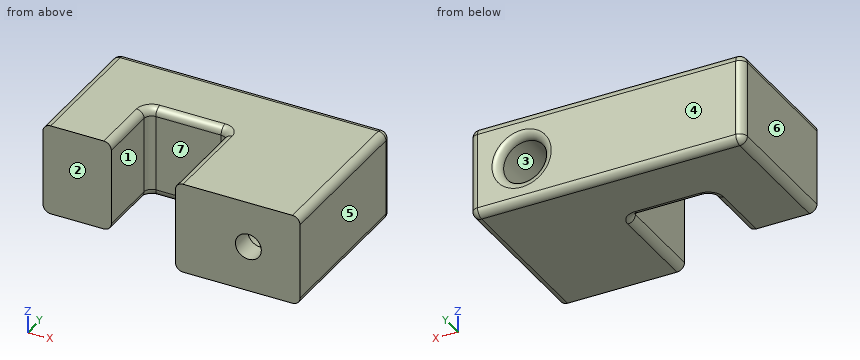
```python
from build123d import *

# Parameters (mm, degrees)
F1_DEPTH = 15.24
F2_R     = 2.159
F3_DEPTH = 27.94
F4_R     = 3.683
F5_DEPTH = 24.13
F6_F1_R  = 1.27
F6_F2_R  = 1.27
F6_F3_R  = 1.27


with BuildPart() as f1:
    # F0 (on Top) → F1 (new body)
    with BuildSketch(Plane.XY):
        Polygon((-11.43, 0), (0, 0), (0, 11.43), (13.462, 11.43), (13.462, -5.08), (34.29, -5.08), (34.29, 22.86), (-11.43, 22.86), align=None)
    extrude(amount=F1_DEPTH)

    # F2 (on face) → F3 (cut, through all)
    with BuildSketch(Plane.XZ.offset(5.08)):
        with Locations((25.654, 7.62)):
            Circle(F2_R)
    extrude(amount=-F3_DEPTH, mode=Mode.SUBTRACT)

    # F4 (on face) → F5 (cut)
    with BuildSketch(Plane(origin=(0, 22.86, 0), x_dir=(-1, 0, 0), z_dir=(0, 1, 0))):
        with Locations((-25.654, 7.62)):
            Circle(F4_R)
    extrude(amount=-F5_DEPTH, mode=Mode.SUBTRACT)

    # F6: fillet of radius 1.27 on 14 edges, made by hand

    # F6_f1
    f6_f1_edges = [f1.edges().sort_by_distance(p)[0] for p in [
        (0, 11.43, 7.62),
        (13.462, 11.43, 7.62),
    ]]
    fillet(f6_f1_edges, radius=F6_F1_R)

    # F6_f2
    f6_f2_edges = [f1.edges().sort_by_distance(p)[0] for p in [
        (6.731, 11.43, 15.24),
        (-11.43, 22.86, 7.62),
        (-11.43, 11.43, 15.24),
        (-11.43, 11.43, 0),
        (11.43, 22.86, 15.24),
        (34.29, 22.86, 7.62),
        (34.29, 8.89, 15.24),
        (34.29, 8.89, 0),
        (11.43, 22.86, 0),
        (29.337, 22.86, 7.62),
        (0.3719743879, 11.0580256121, 15.24),
        (13.0900256121, 11.0580256121, 15.24),
    ]]
    fillet(f6_f2_edges, radius=F6_F2_R)

    # F6_f3
    f6_f3_edges = [f1.edges().sort_by_distance(p)[0] for p in [
        (0, 5.08, 0),
        (6.731, 11.43, 0),
        (0.3719743879, 11.0580256121, 0),
        (13.0900256121, 11.0580256121, 0),
    ]]
    fillet(f6_f3_edges, radius=F6_F3_R)


solid = f1.part
```
Can you work these out from the model? Positions are in its coordinate system, mm. Face numbers are marked on the shaded views. A direction names the side the tool comes from. Round coordinates to 2 decimals unless told otherwise and drop trailing zeros. Loops run counter-clockwise (first coordinate to the right, second up) from the corner with the lowest first, then second, coordinate; pieces in that order, holes last.
Item 1: Please list where these lines run through material, in increasing order: L1, parallel to X at y = 10, z = 11.5; L2, parallel to X at y = 10.75, z = 7.25; L3, parallel to X at y = 2.5, z = 10.
Item 2: Will these pins go through, and if not, where does the flat tip stop? pin 1 Ø3.5 at (x, z) = (8.5, 8) entering from -Y; pin 2 Ø3.5 at (x, z) = (-3, 9) entering from -Y.
Item 3: Which directions (+Z, -Z, +X, -X, +Y, -Y) give clear straight access to the entire face, cutting with the end or side of a thin tool? Please do the marked faces 1, 2 and 3.
Item 4: Suppose I cut it at A-A, the plane z = 7.62. Write out the boundary of the cut face in (x, y) (3 decimals), then the cut area to 3 significant figures.
Item 5: Suppose I cut it at C-C, the plane x = 10. Write out the boundary of the cut face in (y, z).
Item 6: Suppose I cut it at B-B, the plane y = 8.75. Write out the boundary of the cut face in (x, z), then the cut area to 3 significant figures.
Item 7: If we mould it in two halves opening along X, with no side actions, what happens to the marked faces 4, 5, 6 and 7? For each: +X half, -X half, draft (parallel to the pull), parting line (faces both ways), or undercut.
Reported:
1. L1: x = -11.43 to 0, 13.46 to 34.29
1. L2: x = -11.43 to 0.15, 13.32 to 21.99, 29.32 to 34.29
1. L3: x = -11.43 to 0, 13.46 to 22.84, 28.46 to 34.29
2. pin 1: stops at y = 11.43
2. pin 2: stops at y = 0
3. face 1: +Z, -Z, -Y
3. face 2: +Z, -Z, -X, -Y
3. face 3: +Y
4. outline: (-11.43, 0) - (0, 0) - (0, 10.16) arc R1.27 cw to (1.27, 11.43) - (12.192, 11.43) arc R1.27 cw to (13.462, 10.16) - (13.462, -5.08) - (23.495, -5.08) - (23.495, -1.27) - (21.971, -1.27) - (21.971, 21.59) arc R1.27 ccw to (20.701, 22.86) - (-10.16, 22.86) arc R1.27 ccw to (-11.43, 21.59) - close; (27.813, -5.08) - (34.29, -5.08) - (34.29, 21.59) arc R1.27 ccw to (33.02, 22.86) - (30.607, 22.86) arc R1.27 ccw to (29.337, 21.59) - (29.337, -1.27) - (27.813, -1.27) - close
4. area: 802 mm2
5. outline: (11.43, 1.27) arc R1.27 ccw to (12.7, 0) - (21.59, 0) arc R1.27 ccw to (22.86, 1.27) - (22.86, 13.97) arc R1.27 ccw to (21.59, 15.24) - (12.7, 15.24) arc R1.27 ccw to (11.43, 13.97) - close
6. outline: (-11.43, 1.27) arc R1.27 ccw to (-10.16, 0) - (-1.27, 0) arc R1.27 ccw to (0, 1.27) - (0, 13.97) arc R1.27 ccw to (-1.27, 15.24) - (-10.16, 15.24) arc R1.27 ccw to (-11.43, 13.97) - close; (13.46, 1.27) arc R1.27 ccw to (14.73, 0) - (33.02, 0) arc R1.27 ccw to (34.29, 1.27) - (34.29, 13.97) arc R1.27 ccw to (33.02, 15.24) - (14.73, 15.24) arc R1.27 ccw to (13.46, 13.97) - close; hole circle Ø7.37 at (25.65, 7.62)
6. area: 446 mm2
7. face 4: draft
7. face 5: +X half
7. face 6: -X half
7. face 7: undercut
